The listing builds one solid part. Answer for the finished solid, in the listing's coordinates (mm). A direction names the side the tool comes from. Give positions to 0.01 mm unless a question says otherwise; leave off trailing zeros. Write each loop counter-clockwise with the first axis right and the second up, starting at its lowest first coordinate (ties: lowest second). Pieces come first, ordered by that corner, then holes. Notation, with made-up numbers: (47, 66.25) -> (99, 66.25) arc R19 cw to (99, 83.25) -> close; hole circle Ø1 at (-30.5, -6). An arc over 180 degrees is marked (long way). Put each result on its own line as item: value. Start each with the question number.
1) For faces 4 (the flat face through (0, -2, 3)), 5 (the flat face through (10, -3.5, 3)), 6 (the flat face through (0, 0.5, 4)), determine the directions among +Z, -Z, +X, -X, +Y, -Y from which every point of the face is accessible in a straight line to the end or side of a thin tool.
2) Find the intervals of material crossed by line 1 along Y through (x, z) = (-1, 2.45); line 2 along X through (y, z) = (-2.75, 0.55); line 3 along Z through (x, y) = (2.5, 1), in increasing order. Write a range as from..to.
3) A cutting plane is placed at A-A (z = 5.65). Write down the section's boundary in (x, y), then the cut area to 3 significant figures.
4) A cutting plane is placed at C-C (z = 1.2). Write down the section's boundary in (x, y), then the cut area to 4 significant figures.
5) For a pull along Y with two mould halves and no side action, classify faces 1 (the flat face through (-10, -3.5, 3)), 2 (the flat face through (0, 2, 2)), 3 (the flat face through (-9.5, -3, 3)) as released by +Y, released by -Y, zero draft, split by the parting line, or undercut.
6) A cutting plane is placed at B-B (y = 1.75). Write down the section's boundary in (x, z), then the cut area to 3 significant figures.
7) A flat-ended cylindrical pin translates along its axis: pin 1 Ø1.5 at (x, z) = (1, 4.5) entering from -Y. Find the tip coordinate at first contact, or state that the pin passes through.
from build123d import *

# Parameters (mm, degrees)
F0_W     = 22
F0_H     = 7
F1_DEPTH = 6
F2_W     = 20.5
F2_H     = 2
F3_DEPTH = 4
F4_W     = 19
F4_H     = 6
F5_DEPTH = 1.5


with BuildPart() as f1:
    # F0 (on Top) → F1 (new body)
    with BuildSketch(Plane.XY):
        Rectangle(F0_W, F0_H)
    extrude(amount=F1_DEPTH)

    # F2 (on face) → F3 (cut)
    with BuildSketch(Plane.XY.offset(6)):
        with Locations((0, 1.5)):
            Rectangle(F2_W, F2_H)
    extrude(amount=-F3_DEPTH, mode=Mode.SUBTRACT)

    # F4 (on face) → F5 (cut)
    with BuildSketch(Plane.XZ.offset(3.5)):
        with Locations((0, 3)):
            Rectangle(F4_W, F4_H)
    extrude(amount=-F5_DEPTH, mode=Mode.SUBTRACT)


solid = f1.part
Reply:
1. face 4: +Z, -Z, -Y
1. face 5: +Z, -Z, +X, -X, -Y
1. face 6: +Z
2. line 1: y = -2..0.5, 2.5..3.5
2. line 2: x = -11..-9.5, 9.5..11
2. line 3: z = 0..2
3. outline: (-11, -3.5) -> (-9.5, -3.5) -> (-9.5, -2) -> (9.5, -2) -> (9.5, -3.5) -> (11, -3.5) -> (11, 3.5) -> (-11, 3.5) -> close; hole (-10.25, 0.5) -> (10.25, 0.5) -> (10.25, 2.5) -> (-10.25, 2.5) -> close
3. area: 84.5 mm2
4. outline: (-11, -3.5) -> (-9.5, -3.5) -> (-9.5, -2) -> (9.5, -2) -> (9.5, -3.5) -> (11, -3.5) -> (11, 3.5) -> (-11, 3.5) -> close
4. area: 125.5 mm2
5. face 1: released by -Y
5. face 2: undercut
5. face 3: zero draft
6. outline: (-11, 0) -> (11, 0) -> (11, 6) -> (10.25, 6) -> (10.25, 2) -> (-10.25, 2) -> (-10.25, 6) -> (-11, 6) -> close
6. area: 50.0 mm2
7. pin 1: stops at y = -2
